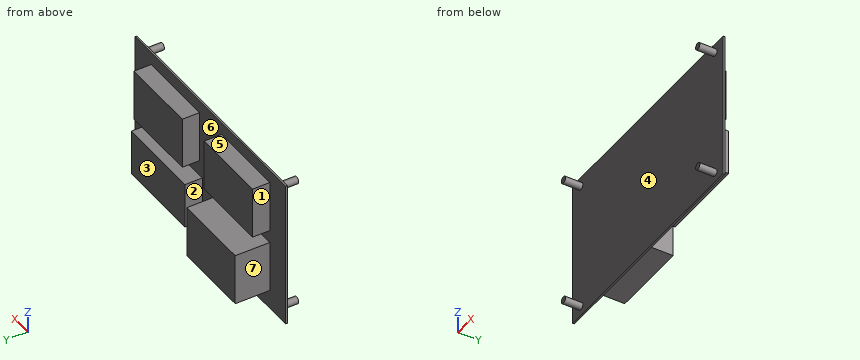
```python
from build123d import *

# Parameters (mm, degrees)
SKETCH_1_W      = 280
SKETCH_1_H      = 172
EXTRUDE_1_DEPTH = 2
SKETCH_2_W      = 90
SKETCH_2_H      = 60
SKETCH_2_W_2    = 100
SKETCH_2_H_2    = 53
EXTRUDE_2_DEPTH = 20
SKETCH_3_W      = 90
SKETCH_3_H      = 60
EXTRUDE_3_DEPTH = 20
SKETCH_4_R      = 4
EXTRUDE_4_DEPTH = 20


with BuildPart() as part:
    # Эскиз1 → Бобышка-Вытянуть1 (new body)
    with BuildSketch(Plane(origin=(0, 0, 0), x_dir=(1, 0, 0), z_dir=(0, 1, 0))):
        Rectangle(SKETCH_1_W, SKETCH_1_H)
    extrude(amount=EXTRUDE_1_DEPTH)

    # Эскиз2 → Бобышка-Вытянуть2 (add)
    with BuildSketch(Plane(origin=(0, 2, 0), x_dir=(1, 0, 0), z_dir=(0, 1, 0))):
        with Locations((-65.639881966, 33.675557069)):
            Rectangle(SKETCH_2_W, SKETCH_2_H)
        with Locations((-65.639881966, -41.201831045)):
            Rectangle(SKETCH_2_W, SKETCH_2_H)
        with Locations((65.116180532, -41.201831045)):
            Rectangle(SKETCH_2_W, SKETCH_2_H)
        with Locations((65.116180532, 33.675557069)):
            Rectangle(SKETCH_2_W_2, SKETCH_2_H_2)
    extrude(amount=EXTRUDE_2_DEPTH)

    # Эскиз3 → Бобышка-Вытянуть3 (add)
    with BuildSketch(Plane(origin=(0, 22, 0), x_dir=(1, 0, 0), z_dir=(0, 1, 0))):
        with Locations((-65.639881966, 33.675557069)):
            Rectangle(SKETCH_3_W, SKETCH_3_H)
    extrude(amount=EXTRUDE_3_DEPTH)

    # Эскиз4 → Бобышка-Вытянуть4 (add)
    with BuildSketch(Plane.XZ):
        with Locations(Location((-125, 75, 0), (0, 0, 270))):
            Circle(SKETCH_4_R)
        with Locations(Location((125, 75, 0), (0, 0, 270))):
            Circle(SKETCH_4_R)
        with Locations(Location((125, -75, 0), (0, 0, 270))):
            Circle(SKETCH_4_R)
        with Locations(Location((-125, -75, 0), (0, 0, 270))):
            Circle(SKETCH_4_R)
    extrude(amount=EXTRUDE_4_DEPTH)


solid = part.part
```
Model file for the job. Use its own axes, mm. Face numbers are marked on the shaded views. A direction names the side the tool comes from. Coordinates: 2 decimals unless noted, no trailing zeros. Order: outer loops, then holes, each group sorted by start corner. A loop starts at its lowest first (then second) coordinate and runs counter-clockwise, first axis right, second up. Notation, with made-up numbers: (-10.75, -22.75) - (-6.75, -22.75) arc R21 cw to (-6.75, 0.25) - close; hole circle Ø5 at (-20, 32). An arc over 180 degrees is marked (long way). Return JSON: item names as keys, results as strings. Group by question number.
1) Saw through at D-D, the plane y = 31.5. Write the cut outline in (x, z), plus the area to 3 significant figures.
2) Saw through at A-A, the plane z = 57.5. Write the cut outline in (x, y), plus the area to 3 significant figures.
3) Saw through at B-B, the plane x = -51. Write the cut outline in (y, z), plus the area to 3 significant figures.
4) Probe line 1 (Z direction, x = 50, y = 3.5); line 2 (Z direction, x = -91.5, y = 11); line 3 (Y direction, x = 90, z = 13). List the from-to ranges inside material, lowest first. Write a range as from..to.
5) Tool access for the marked faces 1, 2, 3 and 4: list every direction of +Z, -Z, +X, -X, +Y, -Y with a clear straight run to the whole face (end or side of a thin tool).
6) Flat gauge pins, fed straight in: P1, Ø1, axis at y = 6, z = 65.5, coming from the +X side; P2, Ø22, axis at y = 17, z = -39, coming from the +X side; P3, Ø20, axis at x = -59.5, y = 25.5, coming from the +Z side; P4, Ø22, axis at y = 8, z = 53.5, coming from the -X side. Where does each tip first touch, or does it go through?
7) Mould opens along X. For the marked faces 5, 6 and 7 say: released by +X, released by -X, zero draft, split by the parting line, or undercut.
8) Saw through at C-C, the plane y = -8.5. Write the cut outline in (x, z).
Values found:
{
 "1": {"outline": "(-110.64, -63.68) - (-20.64, -63.68) - (-20.64, -3.68) - (-110.64, -3.68) - close", "area": "5,400 mm²"},
 "2": {"outline": "(-140, 0) - (140, 0) - (140, 2) - (110.12, 2) - (110.12, 22) - (20.12, 22) - (20.12, 2) - (-20.64, 2) - (-20.64, 22) - (-110.64, 22) - (-110.64, 2) - (-140, 2) - close", "area": "4,160 mm²"},
 "3": {"outline": "(0, -86) - (2, -86) - (2, -63.68) - (42, -63.68) - (42, -3.68) - (2, -3.68) - (2, 11.2) - (22, 11.2) - (22, 71.2) - (2, 71.2) - (2, 86) - (0, 86) - close", "area": "3,940 mm²"},
 "4": {"line 1": "z = -60.18..-7.18, 11.2..71.2", "line 2": "z = -63.68..-3.68, 11.2..71.2", "line 3": "y = 0..22"},
 "5": {"face 1": "+Z, -Z, -X, +Y", "face 2": "+Z, -Z, +Y", "face 3": "+Z, -Z, +X, +Y", "face 4": "-Y"},
 "6": {"P1": "stops at x = 110.12", "P2": "stops at x = 115.12", "P3": "stops at z = 71.2", "P4": "stops at x = -140"},
 "7": {"face 5": "zero draft", "face 6": "undercut", "face 7": "released by -X"},
 "8": {"outline": "circle Ø8 at (-125, -75); circle Ø8 at (-125, 75); circle Ø8 at (125, -75); circle Ø8 at (125, 75)"}
}
